from build123d import *

# Parameters (mm, degrees)
F0_R     = 29.21
F1_DEPTH = 5.08
F2_R     = 1.5875
F3_DEPTH = 25.4


with BuildPart() as f1:
    # F0 (on Front) → F1 (new body)
    with BuildSketch(Plane.XZ):
        Circle(F0_R)
        with BuildLine():
            ThreePointArc((19.147667, 6.802149), (20.024772, 3.451217), (20.32, 0))
            ThreePointArc((20.32, 0), (15.616353, -13.001228), (3.683, -19.983441))
            ThreePointArc((3.683, -19.983441), (1.849173, -20.235685), (0, -20.32))
            ThreePointArc((0, -20.32), (-1.849173, -20.235685), (-3.683, -19.983441))
            ThreePointArc((-3.683, -19.983441), (-17.597636, -10.16), (-19.147667, 6.802149))
            ThreePointArc((-19.147667, 6.802149), (-17.597636, 10.16), (-15.464667, 13.181292))
            ThreePointArc((-15.464667, 13.181292), (0, 20.32), (15.464667, 13.181292))
            ThreePointArc((15.464667, 13.181292), (17.597636, 10.16), (19.147667, 6.802149))
        make_face(mode=Mode.SUBTRACT)
        with BuildLine():
            Line((-3.339771, 6.18098), (-15.464667, 13.181292))
            ThreePointArc((-15.464667, 13.181292), (-17.597636, 10.16), (-19.147667, 6.802149))
            Line((-19.147667, 6.802149), (-7.022771, -0.198163))
            ThreePointArc((-7.022771, -0.198163), (-6.084319, 3.512783), (-3.339771, 6.18098))
        make_face()
        with BuildLine():
            ThreePointArc((3.683, -5.982817), (6.084319, -3.512783), (7.022771, -0.198163))
            ThreePointArc((7.022771, -0.198163), (7.024868, -0.099091), (7.025567, 0))
            ThreePointArc((7.025567, 0), (6.034168, 3.59825), (3.339771, 6.18098))
            ThreePointArc((3.339771, 6.18098), (0, 7.025567), (-3.339771, 6.18098))
            ThreePointArc((-3.339771, 6.18098), (-6.084319, 3.512783), (-7.022771, -0.198163))
            ThreePointArc((-7.022771, -0.198163), (-6.084319, -3.512783), (-3.683, -5.982817))
            ThreePointArc((-3.683, -5.982817), (-1.913885, -6.759854), (0, -7.025567))
            ThreePointArc((0, -7.025567), (1.913885, -6.759854), (3.683, -5.982817))
        make_face()
        with BuildLine():
            ThreePointArc((0, -20.32), (1.849173, -20.235685), (3.683, -19.983441))
            Line((3.683, -19.983441), (3.683, -5.982817))
            ThreePointArc((3.683, -5.982817), (1.913885, -6.759854), (0, -7.025567))
            Line((0, -7.025567), (0, -20.32))
        make_face()
        with BuildLine():
            Line((7.022771, -0.198163), (19.147667, 6.802149))
            ThreePointArc((19.147667, 6.802149), (17.597636, 10.16), (15.464667, 13.181292))
            Line((15.464667, 13.181292), (3.339771, 6.18098))
            ThreePointArc((3.339771, 6.18098), (6.034168, 3.59825), (7.025567, 0))
            ThreePointArc((7.025567, 0), (7.024868, -0.099091), (7.022771, -0.198163))
        make_face()
        with BuildLine():
            ThreePointArc((-3.683, -19.983441), (-1.849173, -20.235685), (0, -20.32))
            Line((0, -20.32), (0, -7.025567))
            ThreePointArc((0, -7.025567), (-1.913885, -6.759854), (-3.683, -5.982817))
            Line((-3.683, -5.982817), (-3.683, -19.983441))
        make_face()
    extrude(amount=F1_DEPTH)

    # F2 (on face) → F3 (cut)
    with BuildSketch(Plane.XZ.offset(5.08)):
        Circle(F2_R)
    extrude(amount=-F3_DEPTH, mode=Mode.SUBTRACT)


solid = f1.part
Work out the finished part from the listing and answer in its coordinate system (mm). A direction names the side the tool comes from. Round coordinates to 2 decimals unless told otherwise and drop trailing zeros. Write each loop counter-clockwise with the first axis right and the second up, starting at its lowest first coordinate (ties: lowest second). Pieces come first, ordered by that corner, then holes. Notation, with made-up numbers: (-28, -22.75) - (2, -22.75) arc R16 ccw to (2, 3.25) - close; hole circle Ø11 at (-12, -8.5). An arc over 180 degrees is marked (long way). Answer in a Markdown table with one row per item. Add a question column.
1. Given pin 1 (1.5 mm diameter, centred on x = 23.5, y = -1, fed in from -Z); pin 2 (2 mm diameter, centred on x = 21.5, y = -1.5, fed in from -Z); pin 3 (1.5 mm diameter, centred on y = -3.5, z = -12.5, fed in from +X); pin 4 (2.5 mm diameter, centred on x = 0, z = 0, fed in from +Y), each flat-ended and moving along its own axis, determine where each tip first touches the part or whether it passes through.
2. Find the intervals of material crossed by line 1 along X through (y, z) = (-4.6, -2.5); line 2 along X through (y, z) = (-2.75, 3); line 3 along Z through (x, y) = (-1, -1.05), in increasing order. Write a range as from..to.
3. The mould has two halves that part along X. Classify faces 1 (the flat face through (-13.17, -2.5, 3.35)), 2 (the cylindrical face through (-21.53, -2.5, 19.74)), 3 (the flat face through (6, -5.08, 0)): +X half, -X half, draft (parallel to the pull), parting line (faces both ways), or undercut.
4. A cutting plane is placed at A-A, the plane x = 0. Determine the outline of the cut face in (y, z), and give its area (3 significant figures).
5. A cutting plane is placed at C-C, the plane x = 17. Determine the outline of the cut face in (y, z), and give its area (3 significant figures).
6. For faces 4 (the flat face through (6, 0, 0)), 5 (the flat face through (9.49, -2.5, 9.73)), determine the directions among +Z, -Z, +X, -X, +Y, -Y from which every point of the face is accessible in a straight line to the end or side of a thin tool.
7. A cutting plane is placed at D-D, the plane z = -22. Determine the outline of the cut face in (x, y).
8. A cutting plane is placed at B-B, the plane y = -4.1. Determine the outline of the cut face in (x, z) (1 decimal).
Worked out:
| question | item | result |
|---|---|---|
| 1 | pin 1 | z = -18.32 |
| 1 | pin 2 | z = -20.81 |
| 1 | pin 3 | x = 26.74 |
| 1 | pin 4 | through |
| 2 | line 1 | -29.1..-20.17, -6.57..6.57, 20.17..29.1 |
| 2 | line 2 | -29.06..-20.1, -12.56..12.56, 20.1..29.06 |
| 2 | line 3 | -29.19..-1.23, 1.23..6.95, 20.3..29.19 |
| 3 | face 1 | undercut |
| 3 | face 2 | parting line |
| 3 | face 3 | draft |
| 4 | outline | (-5.08, -29.21) - (0, -29.21) - (0, -1.59) - (-5.08, -1.59) - close; (-5.08, 1.59) - (0, 1.59) - (0, 7.03) - (-5.08, 7.03) - close; (-5.08, 20.32) - (0, 20.32) - (0, 29.21) - (-5.08, 29.21) - close |
| 4 | area | 213 mm^2 |
| 5 | outline | (-5.08, -23.75) - (0, -23.75) - (0, -11.13) - (-5.08, -11.13) - close; (-5.08, 5.56) - (0, 5.56) - (0, 23.75) - (-5.08, 23.75) - close |
| 5 | area | 157 mm^2 |
| 6 | face 4 | +Z, -Z, +X, -X, +Y |
| 6 | face 5 | +Y, -Y |
| 7 | outline | (-19.22, -5.08) - (19.22, -5.08) - (19.22, 0) - (-19.22, 0) - close |
| 8 | outline | circle Ø58.4 at (0, 0); hole (-19.1, 6.8) arc R20.3 ccw to (-3.7, -20) - (-3.7, -6) arc R7 cw to (-7, -0.2) - close; hole (-15.5, 13.2) - (-3.3, 6.2) arc R7 cw to (3.3, 6.2) - (15.5, 13.2) arc R20.3 ccw to start; hole circle Ø3.2 at (0, 0); hole (3.7, -20) arc R20.3 ccw to (20.3, 0) arc R20.3 ccw to (19.1, 6.8) - (7, -0.2) arc R7 cw to (3.7, -6) - close |
